Verification items for the finished model (mm, model axes). A direction names the side the tool comes from. Coordinates: 2 decimals unless noted, no trailing zeros. Write each loop counter-clockwise with the first axis right and the second up, starting at its lowest first coordinate (ties: lowest second). Pieces come first, ordered by that corner, then holes. Notation, with made-up numbers: (87, 12) - (97, 12) arc R16 ccw to (97, 30) - close; hole circle Ø10 at (74, 42). An arc over 180 degrees is marked (long way). Answer as CSV lines item,"result". Start each with the question number.
```python
from build123d import *

# Parameters (mm, degrees)
SKETCH1_R           = 152.4
SKETCH1_R_2         = 139.7
BOSS_EXTRUDE1_DEPTH = 25.4
SKETCH1_3_R         = 139.7
SKETCH1_3_R_2       = 127
BOSS_EXTRUDE2_DEPTH = 12.7
SKETCH2_W           = 6.35
SKETCH2_H           = 3.175
BOSS_EXTRUDE3_DEPTH = 12.7
CUT_EXTRUDE1_DEPTH  = 25.4
CIRPATTERN1_COUNT   = 4


with BuildPart() as part:
    # Sketch1 → Boss-Extrude1 (new body)
    with BuildSketch(Plane(origin=(0, 0, 0), x_dir=(1, 0, 0), z_dir=(0, 1, 0))):
        with Locations(Location((0, 0, 0), (0, 0, 270))):
            Circle(SKETCH1_R)
        with Locations(Location((0, 0, 0), (0, 0, 270))):
            Circle(SKETCH1_R_2, mode=Mode.SUBTRACT)
    extrude(amount=BOSS_EXTRUDE1_DEPTH)

    # Sketch1_3 → Boss-Extrude2 (add)
    with BuildSketch(Plane(origin=(0, 0, 0), x_dir=(1, 0, 0), z_dir=(0, 1, 0))):
        with Locations(Location((0, 0, 0), (0, 0, 270))):
            Circle(SKETCH1_3_R)
        with Locations(Location((0, 0, 0), (0, 0, 270))):
            Circle(SKETCH1_3_R_2, mode=Mode.SUBTRACT)
    extrude(amount=BOSS_EXTRUDE2_DEPTH)

    # Sketch2 → Boss-Extrude3 (add)
    with BuildSketch(Plane.XZ):
        with BuildLine():
            ThreePointArc((-126.841150657, 6.35), (-127, 0), (-126.841150657, -6.35))
            Line((-126.841150657, -6.35), (-120.491150657, -6.35))
            Line((-120.491150657, -6.35), (-120.491150657, 6.35))
            Line((-120.491150657, 6.35), (-126.841150657, 6.35))
        make_face()
        with BuildLine():
            ThreePointArc((6.35, 126.841150657), (0, 127), (-6.35, 126.841150657))
            Line((-6.35, 126.841150657), (-6.35, 120.491150657))
            Line((-6.35, 120.491150657), (6.35, 120.491150657))
            Line((6.35, 120.491150657), (6.35, 126.841150657))
        make_face()
        with BuildLine():
            Line((120.491150657, -6.35), (126.841150657, -6.35))
            ThreePointArc((126.841150657, -6.35), (126.960281453, -3.175993274), (127, 0))
            ThreePointArc((127, 0), (126.960281453, 3.175993274), (126.841150657, 6.35))
            Line((126.841150657, 6.35), (120.491150657, 6.35))
            Line((120.491150657, 6.35), (120.491150657, -6.35))
        make_face()
        with BuildLine():
            Line((0, -123.666150657), (0, -127))
            ThreePointArc((0, -127), (3.175993274, -126.960281453), (6.35, -126.841150657))
            Line((6.35, -126.841150657), (6.35, -123.666150657))
            Line((6.35, -123.666150657), (0, -123.666150657))
        make_face()
        with Locations((3.175, -122.078650657)):
            Rectangle(SKETCH2_W, SKETCH2_H)
        with Locations((-3.175, -122.078650657)):
            Rectangle(SKETCH2_W, SKETCH2_H)
        with BuildLine():
            ThreePointArc((-6.35, -126.841150657), (-3.175993274, -126.960281453), (0, -127))
            Line((0, -127), (0, -123.666150657))
            Line((0, -123.666150657), (-6.35, -123.666150657))
            Line((-6.35, -123.666150657), (-6.35, -126.841150657))
        make_face()
    extrude(amount=-BOSS_EXTRUDE3_DEPTH)

    # Sketch3 → Cut-Extrude1 (cut)
    with BuildSketch(Plane(origin=(-120.491150657, 0, 0), x_dir=(0, 0, -1), z_dir=(1, 0, 0))):
        with BuildLine():
            ThreePointArc((2, 6.35), (1.414213562, 7.764213562), (0, 8.35))
            Line((0, 8.35), (0, 4.35))
            ThreePointArc((0, 4.35), (1.414213562, 4.935786438), (2, 6.35))
        make_face()
        with BuildLine():
            Line((0, 4.35), (0, 8.35))
            ThreePointArc((0, 8.35), (-2, 6.35), (0, 4.35))
        make_face()
    cut_extrude1 = extrude(amount=-CUT_EXTRUDE1_DEPTH, mode=Mode.SUBTRACT)

    # CirPattern1: Cut-Extrude1 ×4 about axis
    cirpattern1_axis = Axis((0, 12.7, 0), (0, 1, 0))
    for i in range(1, CIRPATTERN1_COUNT):
        add(cut_extrude1.rotate(cirpattern1_axis, i * 360 / CIRPATTERN1_COUNT), mode=Mode.SUBTRACT)


solid = part.part
```
1. Depth check by flat-ended pin: P1, Ø5, axis at y = 14, z = 15.5, coming from the -X side; P2, Ø3, axis at x = 123, y = 4, coming from the +Z side; P3, Ø3, axis at y = 9.5, z = -122, coming from the -X side; P4, Ø4.5, axis at x = 0.5, y = 6, coming from the +Z side. Enter the tip coordinate at first touch or a pass-through.
2. Scan lines: line 1 along X through (y, z) = (18, 0); line 2 along Z through (x, y) = (1.5, 12.5); line 3 along Y through (x, z) = (126.5, 31). Record each from-to range of solid material in increasing order. Write a range as from..to.
3. Cross-section at C-C (y = 17). Record the cut outline in (x, z).
4. Access from +Z, -Z, +X, -X, +Y, -Y to the whole of each face (thin tool, end or side, straight path). Record for faces 1 (the face through (-123, 25.4, 67)), 2 (the face through (-136.38, 18.96, -30.28)), 3 (the face through (-90.722, 6.261, 88.873)).
5. Draft check along Z on faces 4 (the face through (2, 5, -120.491)), 5 (the face through (-92.73, 12.52, -120.94)), 6 (the face through (-1, 0, 125)). Enter one of: pulls with the +Z half, pulls with the -Z half, needs draft (parallel to the pull), parting line crosses it, or undercut.
6. Cross-section at B-B (z = -45). Record the cut outline in (x, y), and give its area (3 significant figures).
7. Cross-section at A-A (x = -94). Record the cut outline in (y, z).
Completed:
1,P1,"stops at x = -151.84"
1,P2,"stops at z = 92"
1,P3,"stops at x = -93.3"
1,P4,"stops at z = 152.4"
2,line 1,"x = -152.4..-139.7, 139.7..152.4"
2,line 2,"z = -152.39..-120.49, 120.49..152.39"
2,line 3,"y = 0..12.7"
3,outline,"circle Ø304.8 at (0, 0); hole circle Ø279.4 at (0, 0)"
4,face 1,"+Z, -Z, +X, -X, +Y"
4,face 2,"+Y"
4,face 3,"+Y, -Y"
5,face 4,"undercut"
5,face 5,"parting line crosses it"
5,face 6,"needs draft"
6,outline,"(-145.6, 0) - (-118.76, 0) - (-118.76, 12.7) - (-132.25, 12.7) - (-132.25, 25.4) - (-145.6, 25.4) - close; (118.76, 0) - (145.6, 0) - (145.6, 25.4) - (132.25, 25.4) - (132.25, 12.7) - (118.76, 12.7) - close"
6,area,"1,020 mm2"
7,outline,"(0, -119.96) - (25.4, -119.96) - (25.4, -103.34) - (12.7, -103.34) - (12.7, -85.4) - (0, -85.4) - close; (0, 85.4) - (12.7, 85.4) - (12.7, 103.34) - (25.4, 103.34) - (25.4, 119.96) - (0, 119.96) - close"
